Source: three-view drawing plus pictorial views. Frame: mm from the lowest corner of the part. A direction names the side the tool comes from. Give positions to 0.01 mm unless a question says otherwise; leave off trailing zeros. Loops run counter-clockwise (first coordinate to the right, second up) from the corner with the lowest first, then second, coordinate; pieces in that order, holes last. Notation, with made-up numbers: (-13.75, 50) -> (36.25, 50) arc R21 cw to (36.25, 65) -> close; hole circle Ø4 at (-25, 58.25). An arc over 180 degrees is marked (long way). Put each result on its own line as item: value.
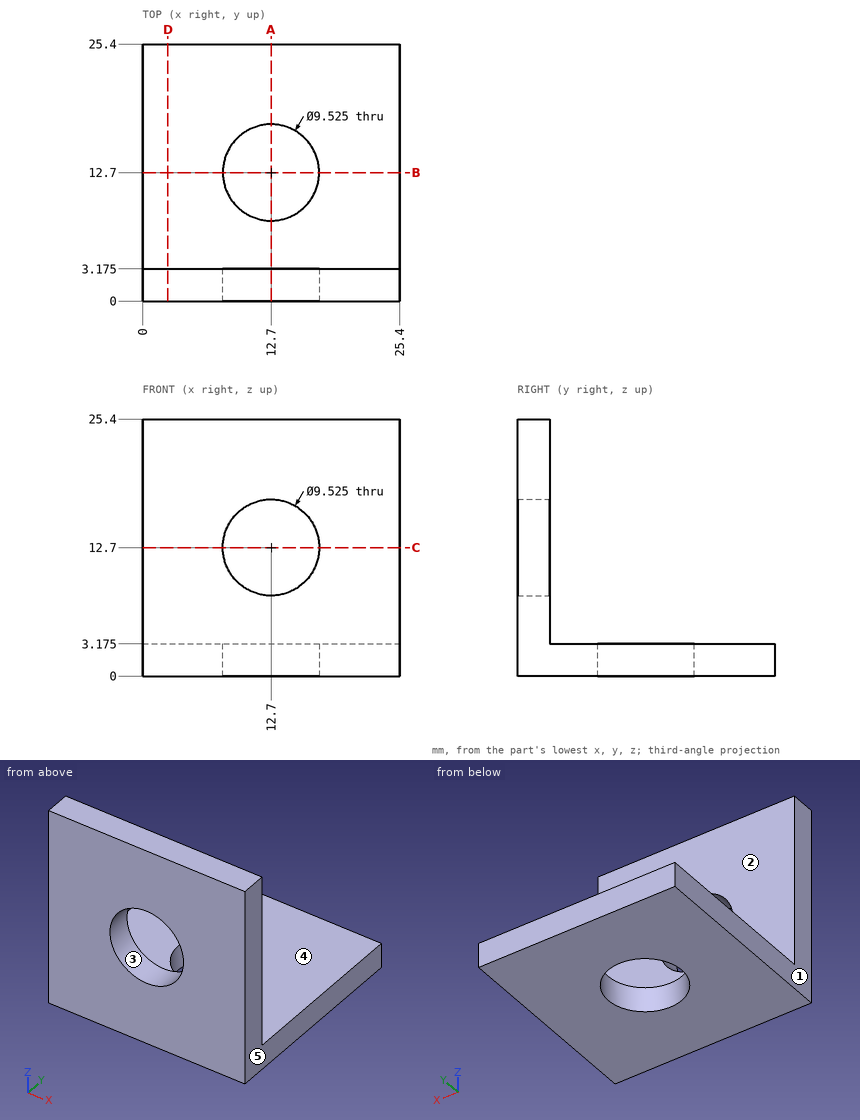
(1) Section A-A on x = 12.7. Return loops of the section in (y, z) (1 decimal).
Calculated:
outline: (0, 0) -> (7.9, 0) -> (7.9, 3.2) -> (3.2, 3.2) -> (3.2, 7.9) -> (0, 7.9) -> close; (0, 17.5) -> (3.2, 17.5) -> (3.2, 25.4) -> (0, 25.4) -> close; (17.5, 0) -> (25.4, 0) -> (25.4, 3.2) -> (17.5, 3.2) -> close
(2) First-contact query: P1, Ø3, axis at x = 17, y = 6, coming from the +Z side (3 decimals); P2, Ø1, axis at x = 8, z = 16, coming from the +Y side (3 decimals). Flat tips, straight axial feed; report the tip coordinate or a pass-through.
Calculated:
P1: stops at z = 3.175
P2: stops at y = 3.175
(3) Reachability of the marked faces 1 and 2 from +Z, -Z, +X, -X, +Y, -Y: full face, straight path, thin tool, end or side. Return the list, or none.
Calculated:
face 1: +Z, -Z, -X, +Y, -Y
face 2: +Z, +X, -X, +Y
(4) Draft query along Z for the marked faces 3, 4 and 5. Return one class per face: released by +Z, released by -Z, zero draft, split by the parting line, or undercut.
Calculated:
face 3: undercut
face 4: released by +Z
face 5: zero draft
(5) Line query: probe 1 along X at (y, z) = (2.1, 12.7). Output: solid intervals per line, ascending. Write a range as from..to.
Calculated:
probe 1: x = 0..7.94, 17.46..25.4
(6) Section D-D on x = 2.5. Return loops of the section in (y, z) (3 decimals).
Calculated:
outline: (0, 0) -> (25.4, 0) -> (25.4, 3.175) -> (3.175, 3.175) -> (3.175, 25.4) -> (0, 25.4) -> close
(7) Section B-B on y = 12.7. Return loops of the section in (x, z) (1 decimal).
Calculated:
outline: (0, 0) -> (7.9, 0) -> (7.9, 3.2) -> (0, 3.2) -> close; (17.5, 0) -> (25.4, 0) -> (25.4, 3.2) -> (17.5, 3.2) -> close
